from build123d import *

# Parameters (mm, degrees)
PAD001_DEPTH = 2


with BuildPart() as part:
    # CopySketch002 → Pad001 (new body)
    with BuildSketch(Plane.XY):
        with BuildLine():
            ThreePointArc((1.361587, 7.37537), (2.17857, 6.704948), (3.233587, 6.76712))
            Line((3.233587, 6.76712), (5.43668, 5.166479))
            ThreePointArc((5.43668, 5.166479), (5.70357, 4.143886), (6.59364, 3.574061))
            Line((6.59364, 3.574061), (7.435147, 0.984169))
            ThreePointArc((7.435147, 0.984169), (7.05, 0), (7.435147, -0.984169))
            Line((7.435147, -0.984169), (6.59364, -3.574061))
            ThreePointArc((6.59364, -3.574061), (5.70357, -4.143886), (5.43668, -5.166479))
            Line((3.233587, -6.76712), (5.43668, -5.166479))
            ThreePointArc((3.233587, -6.76712), (2.17857, -6.704948), (1.361587, -7.37537))
            Line((-1.361587, -7.37537), (1.361587, -7.37537))
            ThreePointArc((-1.361587, -7.37537), (-2.17857, -6.704948), (-3.233587, -6.76712))
            Line((-5.43668, -5.166479), (-3.233587, -6.76712))
            ThreePointArc((-5.43668, -5.166479), (-5.70357, -4.143886), (-6.59364, -3.574061))
            Line((-7.435147, -0.984169), (-6.59364, -3.574061))
            ThreePointArc((-7.435147, -0.984169), (-7.05, 0), (-7.435147, 0.984169))
            Line((-6.59364, 3.574061), (-7.435147, 0.984169))
            ThreePointArc((-6.59364, 3.574061), (-5.70357, 4.143886), (-5.43668, 5.166479))
            Line((-5.43668, 5.166479), (-3.233587, 6.76712))
            ThreePointArc((-3.233587, 6.76712), (-2.17857, 6.704948), (-1.361587, 7.37537))
            Line((-1.361587, 7.37537), (1.361587, 7.37537))
        make_face()
        with BuildLine():
            Line((5.617724, -0.964976), (5.112033, -2.521333))
            ThreePointArc((5.112033, -2.521333), (4.247339, -3.085873), (3.977636, -4.082697))
            Line((3.977636, -4.082697), (2.653719, -5.044579))
            ThreePointArc((2.653719, -5.044579), (1.622339, -4.993047), (0.818226, -5.640967))
            Line((0.818226, -5.640967), (-0.818226, -5.640967))
            ThreePointArc((-0.818226, -5.640967), (-1.622339, -4.993047), (-2.653719, -5.044579))
            Line((-2.653719, -5.044579), (-3.977636, -4.082697))
            ThreePointArc((-3.977636, -4.082697), (-4.247339, -3.085873), (-5.112033, -2.521333))
            Line((-5.112033, -2.521333), (-5.617724, -0.964976))
            ThreePointArc((-5.617724, -0.964976), (-5.25, 0), (-5.617724, 0.964976))
            Line((-5.617724, 0.964976), (-5.112033, 2.521333))
            ThreePointArc((-5.112033, 2.521333), (-4.247339, 3.085873), (-3.977636, 4.082697))
            Line((-3.977636, 4.082697), (-2.653719, 5.044579))
            ThreePointArc((-2.653719, 5.044579), (-1.622339, 4.993047), (-0.818226, 5.640967))
            Line((-0.818226, 5.640967), (0.818226, 5.640967))
            ThreePointArc((0.818226, 5.640967), (1.622339, 4.993047), (2.653719, 5.044579))
            Line((2.653719, 5.044579), (3.977636, 4.082697))
            ThreePointArc((3.977636, 4.082697), (4.247339, 3.085873), (5.112033, 2.521333))
            Line((5.112033, 2.521333), (5.617724, 0.964976))
            ThreePointArc((5.617724, 0.964976), (5.25, 0), (5.617724, -0.964976))
        make_face(mode=Mode.SUBTRACT)
    extrude(amount=PAD001_DEPTH)


solid = part.part
Read the model definition and answer for the solid it produces. Units are mm, in the model's axes. A direction names the side the tool comes from. Give positions to 0.01 mm unless a question says otherwise; leave off trailing zeros. Write each loop counter-clockwise with the first axis right and the second up, starting at its lowest first coordinate (ties: lowest second). Pieces come first, ordered by that corner, then holes. Notation, with made-up numbers: (-7.5, 28.25) - (19.5, 28.25) arc R32 ccw to (19.5, 56.25) - close; hole circle Ø2 at (-35, -6.5). An arc over 180 degrees is marked (long way). Use CSV: the item, a comma, the result in double quotes. Start each with the question number.
Item 1: The part is cut by section B-B, the plane x = 3. Give the vertices of the cut face in (y, z), and give its area (3 significant figures).
Item 2: For faces 4 (the flat face through (-3.32, 4.56, 0.99)), 5 (the flat face through (7.009, 2.297, 0.986)), determine the directions among +Z, -Z, +X, -X, +Y, -Y from which every point of the face is accessible in a straight line to the end or side of a thin tool.
Item 3: A flat-ended cylindrical pin translates along its axis: P1, Ø1, axis at y = -2.5, z = 0.5, coming from the -X side. Find the tip coordinate at first contact, or state that the pin passes through.
Item 4: The part is cut by section A-A, the plane y = 0. Give the vertices of the cut face in (x, z), and give its area (3 significant figures).
Item 5: The part is cut by section C-C, the plane x = -6.25. Give the vertices of the cut face in (y, z), and give its area (3 significant figures).
Item 6: Consider line 1 (X direction, y = 5.25, z = 1.55); line 2 (Y direction, x = -0.75, z = 0.9); line 3 (X direction, y = -3.5, z = 0.2). Determine where each line is inside the solid, lowest interval first.
Item 7: The mould has two halves that part along X. Classify faces 1 (the flat face through (-7.009, 2.297, 0.986)), 2 (the flat face through (-5, 3, 2)), 3 (the cylindrical face through (1.6, -5, 1)): pulls with the +X half, pulls with the -X half, needs draft (parallel to the pull), parting line crosses it, or undercut.
Taken from the geometry:
1,outline,"(-6.68, 0) - (-4.79, 0) - (-4.79, 2) - (-6.68, 2) - close; (4.79, 0) - (6.68, 0) - (6.68, 2) - (4.79, 2) - close"
1,area,"7.56 mm2"
2,face 4,"+Z, -Z"
2,face 5,"+Z, -Z, +X, +Y"
3,P1,"x = -7.11"
4,outline,"(-7.05, 0) - (-5.25, 0) - (-5.25, 2) - (-7.05, 2) - close; (5.25, 0) - (7.05, 0) - (7.05, 2) - (5.25, 2) - close"
4,area,"7.20 mm2"
5,outline,"(-3.69, 0) - (3.69, 0) - (3.69, 2) - (-3.69, 2) - close"
5,area,"14.8 mm2"
6,line 1,"-5.32 to -1.15, 1.15 to 5.32"
6,line 2,"-7.38 to -5.64, 5.64 to 7.38"
6,line 3,"-6.62 to -4.04, 4.04 to 6.62"
7,face 1,"pulls with the -X half"
7,face 2,"needs draft"
7,face 3,"undercut"
